from build123d import *

# Parameters (mm, degrees)
SKETCH019_R      = 1.5
EXTRUDE022_DEPTH = 4
SKETCH020_R      = 2.5
EXTRUDE020_DEPTH = 4
SKETCH022_W      = 90.25
SKETCH022_H      = 53.1
EXTRUDE019_DEPTH = 1
SKETCH038_R      = 1.5
EXTRUDE038_DEPTH = 13
SKETCH021_W      = 90.25
SKETCH021_H      = 53.1
EXTRUDE021_DEPTH = 15


with BuildPart() as extrude_mainboardcase_holes:
    # Sketch019 → Extrude022 (new body)
    with BuildSketch(Plane.XY):
        with Locations((3, 42.1)):
            Circle(SKETCH019_R)
        with Locations((3, 3)):
            Circle(SKETCH019_R)
        with Locations((79.25, 42.1)):
            Circle(SKETCH019_R)
        with Locations((79.25, 3)):
            Circle(SKETCH019_R)
    extrude(amount=EXTRUDE022_DEPTH)


with BuildPart() as extrude_mainboardcase_holes_1:
    # Extrude022 placement: moved
    add(extrude_mainboardcase_holes.part.moved(Location((0, 0, 1))))


with BuildPart() as obj1:
    # Sketch020 → Extrude020 (new body)
    with BuildSketch(Plane.XY):
        with Locations((3, 42.1)):
            Circle(SKETCH020_R)
        with Locations((79.25, 3)):
            Circle(SKETCH020_R)
        with Locations((79.25, 42.1)):
            Circle(SKETCH020_R)
        with Locations((3, 3)):
            Circle(SKETCH020_R)
    extrude(amount=EXTRUDE020_DEPTH)


with BuildPart() as obj1_1:
    # Extrude020 placement: moved
    add(obj1.part.moved(Location((0, 0, 1))))

    # Cut: cut Extrude_MainBoardCase_holes
    add(extrude_mainboardcase_holes_1.part, mode=Mode.SUBTRACT)


with BuildPart() as extrude_mainboardcase_bottom:
    # Sketch022 → Extrude019 (new body)
    with BuildSketch(Plane.XY):
        with Locations((41.125, 22.55)):
            Rectangle(SKETCH022_W, SKETCH022_H)
    extrude(amount=EXTRUDE019_DEPTH)


with BuildPart() as extrude038:
    # Sketch038 → Extrude038 (new body)
    with BuildSketch(Plane.XY):
        with Locations((-1.9, 47)):
            Circle(SKETCH038_R)
        with Locations((84.15, 47)):
            Circle(SKETCH038_R)
        with Locations((-1.9, -1.9)):
            Circle(SKETCH038_R)
        with Locations((84.15, -1.9)):
            Circle(SKETCH038_R)
    extrude(amount=EXTRUDE038_DEPTH)


with BuildPart() as extrude038_1:
    # Extrude038 placement: moved
    add(extrude038.part.moved(Location((0, 0, 2))))


with BuildPart() as fusion_mainboardcase_bottom:
    # Sketch021 → Extrude021 (new body)
    with BuildSketch(Plane.XY):
        with Locations((41.125, 22.55)):
            Rectangle(SKETCH021_W, SKETCH021_H)
        Polygon((1, 47.1), (81.25, 47.1), (84.25, 44.1), (84.25, 1), (81.25, -2), (1, -2), (-2, 1), (-2, 44.1), align=None, mode=Mode.SUBTRACT)
    extrude(amount=EXTRUDE021_DEPTH)

    # Cut009: cut Extrude038
    add(extrude038_1.part, mode=Mode.SUBTRACT)

    # Fusion011: union obj1, Extrude_MainBoardCase_Bottom
    add(obj1_1.part)
    add(extrude_mainboardcase_bottom.part)


solid = fusion_mainboardcase_bottom.part
Design review of the part built by this model. Coordinates are the model's own, in mm. Give positions to 0.01 mm unless a question says otherwise; leave off trailing zeros. Loops run counter-clockwise (first coordinate to the right, second up) from the corner with the lowest first, then second, coordinate; pieces in that order, holes last. Notation, with made-up numbers: (20, -21.5) -> (33, -21.5) arc R25 cw to (33, 5.5) -> close; hole circle Ø3 at (17.5, 38.5). An arc over 180 degrees is marked (long way). One line per question, with ' | ' between items. Start each with the question number.
(1) We need section C-C (z = 13.75). State the section outline as (x, y) points.
(2) We need section B-B (x = 70). State the section outline as (y, z) points.
(3) We need section A-A (y = 3). State the section outline as (x, z) points.
(4) We need section D-D (y = 31). State the section outline as (x, z) points, and give its area (3 significant figures).
(5) Insertion check: P1, Ø3.5, axis at x = 3.5, y = 42.5, coming from the +Z side; P2, Ø2.5, axis at x = 84.15, y = -1.9, coming from the +Z side; P3, Ø3.5, axis at x = 84.15, y = 47, coming from the -Z side. Each pin has a flat end and moves straight along its axis. Give the tip position at first contact, or say it passes through.
(6) For line 1 (Y direction, x = 79.25, z = 3.8); line 2 (X direction, y = 17, z = 11.5); line 3 (Y direction, x = 3.5, z = 7.25), list the stretches that pass through material, from the lowest coordinate up.
(7) Draft analysis for pull direction Y (two halves, no side actions). For faces 1 (the face through (77.266, 1.479, 2.972)), 2 (the face through (-2, -2, 2)), 3 (the face through (86.25, 22, 7)), 4 (the face through (40, 49.1, 7)), state which applies: +Y half, -Y half, draft (parallel to the pull), parting line (faces both ways), or undercut.
The answers:
1) outline: (-4, -4) -> (86.25, -4) -> (86.25, 49.1) -> (-4, 49.1) -> close; hole circle Ø3 at (-1.9, -1.9); hole circle Ø3 at (-1.9, 47); hole (-2, 1) -> (1, -2) -> (81.25, -2) -> (84.25, 1) -> (84.25, 44.1) -> (81.25, 47.1) -> (1, 47.1) -> (-2, 44.1) -> close; hole circle Ø3 at (84.15, -1.9); hole circle Ø3 at (84.15, 47)
2) outline: (-4, 0) -> (49.1, 0) -> (49.1, 15) -> (47.1, 15) -> (47.1, 1) -> (-2, 1) -> (-2, 15) -> (-4, 15) -> close
3) outline: (-4, 0) -> (86.25, 0) -> (86.25, 15) -> (84.25, 15) -> (84.25, 1) -> (81.75, 1) -> (81.75, 5) -> (80.75, 5) -> (80.75, 1) -> (77.75, 1) -> (77.75, 5) -> (76.75, 5) -> (76.75, 1) -> (5.5, 1) -> (5.5, 5) -> (4.5, 5) -> (4.5, 1) -> (1.5, 1) -> (1.5, 5) -> (0.5, 5) -> (0.5, 1) -> (-2, 1) -> (-2, 15) -> (-4, 15) -> close
4) outline: (-4, 0) -> (86.25, 0) -> (86.25, 15) -> (84.25, 15) -> (84.25, 1) -> (-2, 1) -> (-2, 15) -> (-4, 15) -> close | area: 146 mm^2
5) P1: stops at z = 5 | P2: stops at z = 2 | P3: stops at z = 0
6) line 1: y = -4 to -2, 0.5 to 1.5, 4.5 to 5.5, 39.6 to 40.6, 43.6 to 44.6, 47.1 to 49.1 | line 2: x = -4 to -2, 84.25 to 86.25 | line 3: y = -4 to -2, 47.1 to 49.1
7) face 1: undercut | face 2: undercut | face 3: draft | face 4: +Y half
